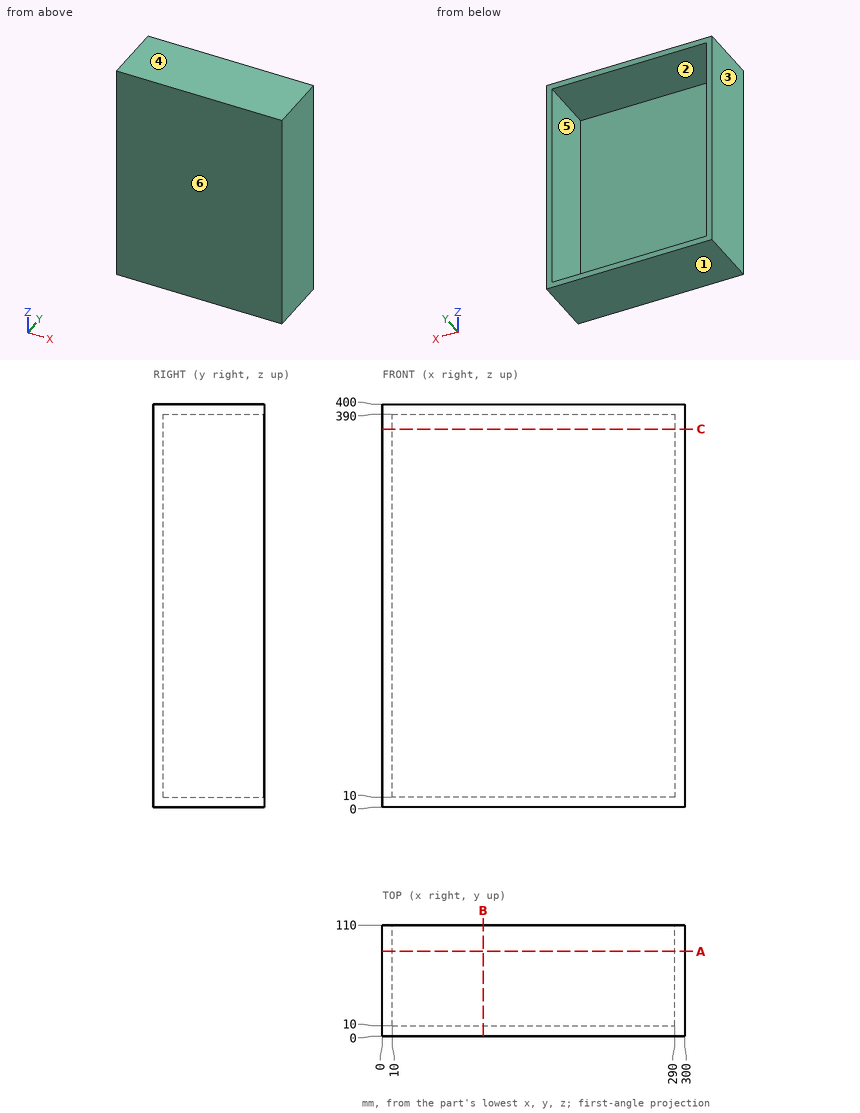
Print and shaded views of the part. All mm, measured from the part's lowest x, y and z. A direction names the side the tool comes from. Coordinates: 2 decimals unless noted, no trailing zeros. Order: outer loops, then holes, each group sorted by start corner. A loop starts at its lowest first (then second) coordinate and runs counter-clockwise, first axis right, second up.
Item 1: Saw through at B-B on x = 100. List the corners of the cut face in (y, z), then the cut area to 3 significant figures.
Filled in:
outline: (0, 0) - (110, 0) - (110, 10) - (10, 10) - (10, 390) - (110, 390) - (110, 400) - (0, 400) - close
area: 6,000 mm2
Item 2: Drop a flat-ended pin along its axis: pin 1 Ø4 at (x, z) = (266, 94.5) entering from +Y. Give the stop position or say it passes through.
Filled in:
pin 1: stops at y = 10
Item 3: Saw through at A-A on y = 84. List the corners of the cut face in (x, z).
Filled in:
outline: (0, 0) - (300, 0) - (300, 400) - (0, 400) - close; hole (10, 10) - (290, 10) - (290, 390) - (10, 390) - close
Item 4: Saw through at C-C on z = 375. List the corners of the cut face in (x, y).
Filled in:
outline: (0, 0) - (300, 0) - (300, 110) - (290, 110) - (290, 10) - (10, 10) - (10, 110) - (0, 110) - close
Item 5: Tool access for the marked faces 5 and 6: list every direction of +Z, -Z, +X, -X, +Y, -Y with a clear straight run to the whole face (end or side of a thin tool).
Filled in:
face 5: +Y
face 6: +Z, -Z, +X, -X, -Y
Item 6: Drill centre lines: L1, parallel to X at y = 56, z = 302; L2, parallel to Z at x = 168.5, y = 61; L3, parallel to Y at x = 68.5, z = 180. Where is each one in solid material? Low to high.
Filled in:
L1: x = 0 to 10, 290 to 300
L2: z = 0 to 10, 390 to 400
L3: y = 0 to 10
Item 7: Mould opens along Z. For the marked faces 1, 2, 3 and 4 say: released by +Z, released by -Z, zero draft, split by the parting line, or undercut.
Filled in:
face 1: released by -Z
face 2: undercut
face 3: zero draft
face 4: released by +Z
